Design review of the part built by this model. Coordinates are the model's own, in mm. A direction names the side the tool comes from. Give positions to 0.01 mm unless a question says otherwise; leave off trailing zeros. Order: outer loops, then holes, each group sorted by start corner. A loop starts at its lowest first (then second) coordinate and runs counter-clockwise, first axis right, second up. Notation, with made-up numbers: (70, -30.75) - (111, -30.75) arc R10 ccw to (111, -25.75) - close; hole circle Ø2 at (-11, -27). An arc over 180 degrees is marked (long way). Write each question's results on one line, items separated by ' | '. Start each with the question number.
```python
from build123d import *

# Parameters (mm, degrees)
SKETCH_2_W                  = 93.1
SKETCH_2_H                  = 10
EXTRUDE_1_DEPTH             = 3.5
SKETCH_4_W                  = 93.1
SKETCH_4_H                  = 6.5
EXTRUDE_2_DEPTH             = 1.1
SKETCH_5_W                  = 93.1
SKETCH_5_H                  = 10
EXTRUDE_3_DEPTH             = 2
CUT_EXTRUDE_1_DEPTH         = 94.867832616
SKETCH_7_W                  = 83.1
SKETCH_7_H                  = 1.1
EXTRUDE_4_DEPTH             = 3.5
CHAMFER_1_SIZE              = 0.4
CUT_EXTRUDE_2_REACH         = 95.868
SKETCH_8_R                  = 150
SKETCH_9_W                  = 93.1
SKETCH_9_H                  = 2
EXTRUDE_5_DEPTH             = 5
EXTRUDE_5_DIRECTION_2_REACH = 95.868


with BuildPart() as part:
    # 草图2 → 凸台-拉伸1 (new body)
    with BuildSketch(Plane(origin=(0, 0, 0), x_dir=(1, 0, 0), z_dir=(0, 1, 0))):
        with Locations((46.55, 5)):
            Rectangle(SKETCH_2_W, SKETCH_2_H)
    extrude(amount=EXTRUDE_1_DEPTH)

    # 草图4 → 凸台-拉伸2 (add)
    with BuildSketch(Plane(origin=(0, 3.5, 0), x_dir=(1, 0, 0), z_dir=(0, 1, 0))):
        with Locations((46.55, 6.75)):
            Rectangle(SKETCH_4_W, SKETCH_4_H)
    extrude(amount=EXTRUDE_2_DEPTH)

    # 草图5 → 凸台-拉伸3 (add)
    with BuildSketch(Plane(origin=(0, 4.6, 0), x_dir=(1, 0, 0), z_dir=(0, 1, 0))):
        with Locations((46.55, 5)):
            Rectangle(SKETCH_5_W, SKETCH_5_H)
    extrude(amount=EXTRUDE_3_DEPTH)

    # 草图6 → 切除-拉伸1 (cut, through all)
    with BuildSketch(Plane.ZY):
        Polygon((-10, 0), (-6.189488223, 6.6), (-10, 6.6), align=None)
    extrude(amount=-CUT_EXTRUDE_1_DEPTH, mode=Mode.SUBTRACT)

    # 草图7 → 凸台-拉伸4 (add)
    with BuildSketch(Plane.XY.offset(-3.5)):
        with Locations((46.55, 4.05)):
            Rectangle(SKETCH_7_W, SKETCH_7_H)
    extrude(amount=EXTRUDE_4_DEPTH)

    # 倒角1
    chamfer_1_edges = [part.edges().sort_by_distance(p)[0] for p in [
        (90.6, 3.5, 0),
        (2.5, 3.5, 0),
    ]]
    chamfer(chamfer_1_edges, length=CHAMFER_1_SIZE)

    # 草图8 → 切除-拉伸2 (cut, up to next)
    with BuildSketch(Plane.XZ, mode=Mode.PRIVATE) as cut_extrude_2_sk1:
        with Locations((46.55, 147)):
            Circle(SKETCH_8_R)
    cut_extrude_2_tool1 = extrude(cut_extrude_2_sk1.sketch, amount=-CUT_EXTRUDE_2_REACH, mode=Mode.PRIVATE) & part.part
    add(cut_extrude_2_tool1.solids().sort_by_distance((46.55, 0, 147))[0], mode=Mode.SUBTRACT)

    # 草图9 → 凸台-拉伸5 (add)
    with BuildSketch(Plane.XY):
        with Locations((46.55, 5.6)):
            Rectangle(SKETCH_9_W, SKETCH_9_H)
    extrude(amount=EXTRUDE_5_DEPTH)

    # 草图9 → 凸台-拉伸5 direction 2 (add, up to next)
    with BuildSketch(Plane.XY, mode=Mode.PRIVATE) as extrude_5_direction_2_sk1:
        with Locations((46.55, 5.6)):
            Rectangle(SKETCH_9_W, SKETCH_9_H)
    extrude_5_direction_2_tool1 = extrude(extrude_5_direction_2_sk1.sketch, amount=-EXTRUDE_5_DIRECTION_2_REACH, mode=Mode.PRIVATE) - part.part
    add(extrude_5_direction_2_tool1.solids().sort_by_distance((46.55, 5.6, 0))[0])


solid = part.part
```
Q1. Draft analysis for pull direction X (two halves, no side actions). For faces 1 (the flat face through (85, 2, 0)), 2 (the flat face through (5, 4, -2)), 3 (the cylindrical face through (46, 2, -3)), 4 (the flat face through (93.1, 3, -3)), state which applies: pulls with the +X half, pulls with the -X half, needs draft (parallel to the pull), parting line crosses it, or undercut.
Q2. Add section D-D (z = 2.25). Give the boundary of the cut face in (x, y), plus the area to 3 significant figures.
Q3. Machinability: for faces 5 (the flat face through (2, 3.5, -2)), 6 (the flat face through (8, 2, 0)), 7 (the flat face through (0, 3, -3)), 8 (the flat face through (91, 3.5, -2)), which of the approach directions +Z, -Z, +X, -X, +Y, -Y give a long, thin tool a straight path to every point of the face, cutting with its end or side? Answer none if there is none.
Q4. Add section C-C (y = 1.25). Give the boundary of the cut face in (x, z), plus the area to 3 significant figures.
Q5. For line 1 (Y direction, x = 56, z = 4.5); line 2 (Z direction, x = 17, y = 1.75); line 3 (Z direction, x = 83, y = 2.75), list the stretches that pass through material, from the lowest coordinate up. Write a range as [from, to].
Q6. Add section A-A (x = 13.5). Give the boundary of the cut face in (y, z), plus the area to 3 significant figures.
Q7. Insertion check: pin 1 Ø0.8 at (y, z) = (4, -2) entering from -X; pin 2 Ø4 at (x, z) = (46.5, 0.5) entering from -Y; pin 3 Ø1.2 at (x, y) = (3.5, 4.5) entering from +Z; pin 4 Ø3.5 at (x, y) = (10, 2) entering from +Z. Each pin has a flat end and moves straight along its axis. Give the tip position at first contact, or say it passes through.
Verdict:
1) face 1: needs draft | face 2: pulls with the -X half | face 3: undercut | face 4: pulls with the +X half
2) outline: (0, 4.6) - (93.1, 4.6) - (93.1, 6.6) - (0, 6.6) - close | area: 186 mm2
3) face 5: +Z, -X | face 6: +Z, +X, -X, -Y | face 7: +Z, -Z, -X, +Y, -Y | face 8: +Z, +X
4) outline: (0, -9.28) - (93.1, -9.28) - (93.1, 0) - (76.4, 0) arc R150 cw to (16.7, 0) - (0, 0) - close | area: 744 mm2
5) line 1: y = [4.6, 6.6] | line 2: z = [-8.99, -0.06] | line 3: z = [-8.41, 0]
6) outline: (0, -10) - (6.6, -6.19) - (6.6, 5) - (4.6, 5) - (4.6, 0) - (0, 0) - close | area: 63.4 mm2
7) pin 1: stops at x = 5 | pin 2: stops at y = 4.6 | pin 3: stops at z = 5 | pin 4: stops at z = 0
